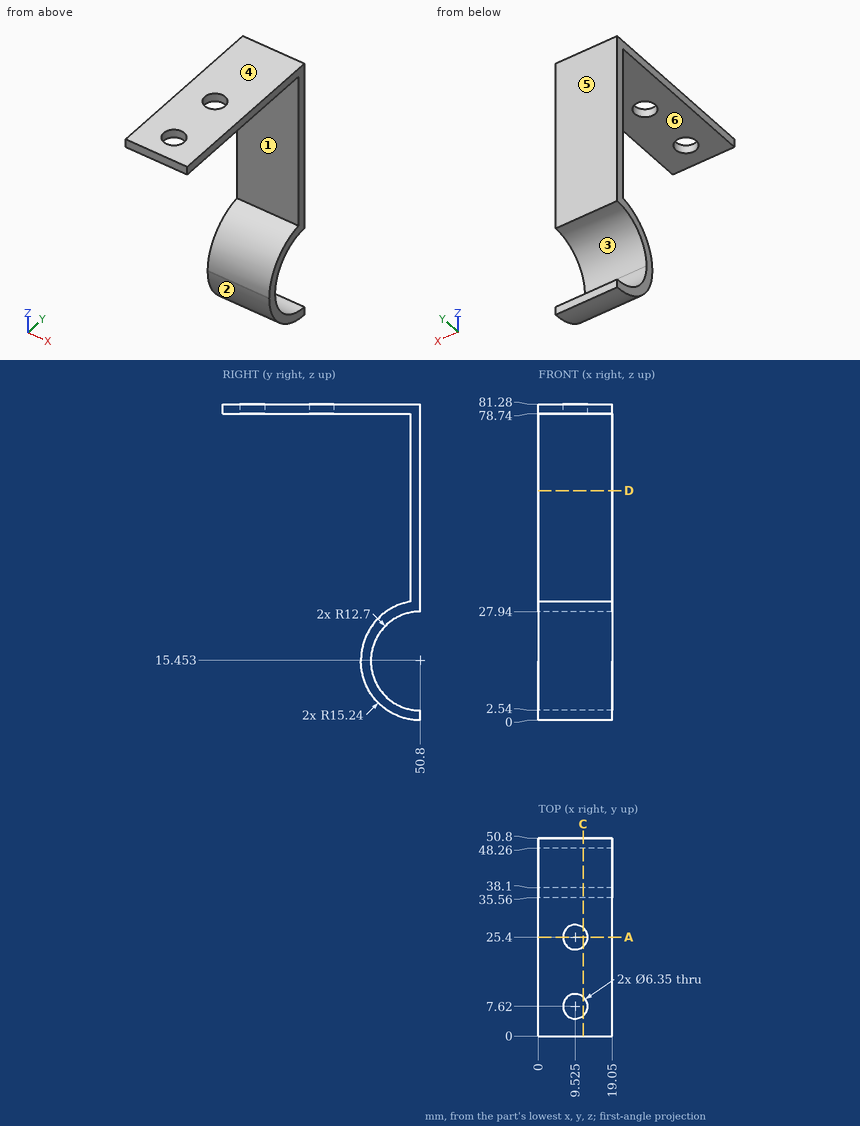
For this review, use the dimensioned drawing (mm, ordinates from the lowest corner) and the shaded views. A direction names the side the tool comes from. Give positions to 0.01 mm unless a question says otherwise; leave off trailing zeros. Order: outer loops, then holes, each group sorted by start corner. A loop starts at its lowest first (then second) coordinate and runs counter-clockwise, first axis right, second up. Notation, with made-up numbers: (8.25, -4.75) - (25.25, -4.75) arc R3 cw to (25.25, 0.25) - close; hole circle Ø6 at (57, 17). An arc over 180 degrees is marked (long way). Use a Markdown table: item, result. Add a question column.
(1) Wall thickness on probe 1 along Z at (x, y) = (7.5, 46.5); probe 2 along Y at (x, z) = (7.25, 47); probe 3 along Z at (x, y) = (11, 12.5): over which ranges is each line inside the solid? List them lowest first. Write a range as [from, to].
(2) Add section A-A on y = 25.4. Give the boundary of the cut face in (x, z).
(3) Add section D-D on z = 59. Give the boundary of the cut face in (x, y), then the cut area to 3 significant figures.
(4) Add section C-C on x = 11.5. Give the number of separate pieces and of enclosed holes in the cut face, then the cut area to 3 significant figures.
(5) Mouldability with a two-part tool opening along Z and no side actions: class the marked faces 4, 5 and 6 as +Z half, -Z half, draft (parallel to the pull), parting line (faces both ways), or undercut.
(6) Machinability: for the marked faces 1, 2 and 3, which of the approach directions +Z, -Z, +X, -X, +Y, -Y give a long, thin tool a straight path to every point of the face, cutting with its end or side? Answer none if there is none.
(7) Clearance check with flat-ended pins moving along their axes: P1, Ø1.5, axis at x = 8.5, z = 27.5, coming from the -Y side; P2, Ø5, axis at x = 9.525, y = 7.62, coming from the +Z side; P3, Ø5.5, axis at x = 10, z = 61.5, coming from the -Y side. State where each tip first meets the part, or that it passes through.
Report:
| question | item | result |
|---|---|---|
| 1 | probe 1 | z = [0.62, 3.29], [27.19, 30.07], [78.74, 81.28] |
| 1 | probe 2 | y = [48.26, 50.8] |
| 1 | probe 3 | z = [78.74, 81.28] |
| 2 | outline | (0, 78.74) - (6.35, 78.74) - (6.35, 81.28) - (0, 81.28) - close; (12.7, 78.74) - (19.05, 78.74) - (19.05, 81.28) - (12.7, 81.28) - close |
| 3 | outline | (0, 48.26) - (19.05, 48.26) - (19.05, 50.8) - (0, 50.8) - close |
| 3 | area | 48.4 mm² |
| 4 | separate pieces | 3 |
| 4 | enclosed holes | 0 |
| 4 | area | 341 mm² |
| 5 | face 4 | +Z half |
| 5 | face 5 | draft |
| 5 | face 6 | undercut |
| 6 | face 1 | +X, -X, -Y |
| 6 | face 2 | -Z, +X, -X, -Y |
| 6 | face 3 | +X, -X, +Y |
| 7 | P1 | stops at y = 40.57 |
| 7 | P2 | passes through |
| 7 | P3 | stops at y = 48.26 |
